```python
from build123d import *

# Parameters (mm, degrees)
F0_W             = 81.28
F0_H             = 58.42
F1_DEPTH         = 3.81
F2_T             = -1.524
F4_DEPTH         = 6.096
F4_COPIES2_COUNT = 2
F6_D             = 1.5113
F6_DEPTH         = 4.826
F6_TIP           = 0.4540403268
F7_R             = 0.635


# Not quite as in the source:
# - a pattern or mirror of a feature is missing from the dataset's text; its kind, count and spacing are read off the source's solid


with BuildPart() as f1:
    # F0 (on Top) → F1 (new body, symmetric)
    with BuildSketch(Plane.XY):
        Rectangle(F0_W, F0_H)
    extrude(amount=F1_DEPTH, both=True)

    # F2
    f2_openings = [f1.faces().sort_by_distance(p)[0] for p in [
        (0, 0, 3.81),
    ]]
    offset(amount=F2_T, openings=f2_openings)

    # F3 (on face) → F4 (join, through all)
    with BuildSketch(Plane.XY.offset(3.81)):
        with BuildLine():
            ThreePointArc((-39.116, 26.162), (-38.0383692655, 26.6083692655), (-37.592, 27.686))
            Line((-37.592, 27.686), (-39.116, 27.686))
            Line((-39.116, 27.686), (-39.116, 26.162))
        make_face()
        with BuildLine():
            ThreePointArc((-13.0386666835, 29.21), (-14.1162974072, 28.7636307286), (-14.5626666667, 27.686))
            Line((-14.5626666667, 27.686), (-11.5146666667, 27.686))
            ThreePointArc((-11.5146666667, 27.686), (-11.9610359381, 28.7636307405), (-13.0386666835, 29.21))
        make_face()
        with BuildLine():
            Line((-39.116, -1.524), (-39.116, 1.524))
            ThreePointArc((-39.116, 1.524), (-40.1936307323, 1.0776307368), (-40.64, 6.4e-09))
            ThreePointArc((-40.64, 6.4e-09), (-40.1936307368, -1.0776307323), (-39.116, -1.524))
        make_face()
        with BuildLine():
            ThreePointArc((14.5626666667, 27.686), (14.1162974012, 28.7636307345), (13.0386666667, 29.21))
            ThreePointArc((13.0386666667, 29.21), (11.9610359321, 28.7636307345), (11.5146666667, 27.686))
            Line((11.5146666667, 27.686), (14.5626666667, 27.686))
        make_face()
        with BuildLine():
            Line((14.5626666667, 27.686), (11.5146666667, 27.686))
            ThreePointArc((11.5146666667, 27.686), (13.0386666667, 26.162), (14.5626666667, 27.686))
        make_face()
        with BuildLine():
            ThreePointArc((-37.592, -27.686), (-38.0383692655, -26.6083692655), (-39.116, -26.162))
            Line((-39.116, -26.162), (-39.116, -27.686))
            Line((-39.116, -27.686), (-37.592, -27.686))
        make_face()
        with BuildLine():
            Line((39.116, 27.686), (37.592, 27.686))
            ThreePointArc((37.592, 27.686), (38.0383692655, 26.6083692655), (39.116, 26.162))
            Line((39.116, 26.162), (39.116, 27.686))
        make_face()
        with BuildLine():
            ThreePointArc((-14.5626666667, -27.686), (-14.1162973989, -28.7636307368), (-13.0386666602, -29.21))
            ThreePointArc((-13.0386666602, -29.21), (-11.9610359299, -28.7636307323), (-11.5146666667, -27.686))
            Line((-11.5146666667, -27.686), (-14.5626666667, -27.686))
        make_face()
        with BuildLine():
            ThreePointArc((11.5146666667, -27.686), (11.9610359295, -28.7636307319), (13.0386666593, -29.21))
            ThreePointArc((13.0386666593, -29.21), (14.1162973986, -28.7636307371), (14.5626666667, -27.686))
            Line((14.5626666667, -27.686), (11.5146666667, -27.686))
        make_face()
        with BuildLine():
            Line((39.116, -1.524), (39.116, 1.524))
            ThreePointArc((39.116, 1.524), (37.592, 0), (39.116, -1.524))
        make_face()
        with BuildLine():
            Line((39.116, -27.686), (39.116, -26.162))
            ThreePointArc((39.116, -26.162), (38.0383692655, -26.6083692655), (37.592, -27.686))
            Line((37.592, -27.686), (39.116, -27.686))
        make_face()
    f4 = extrude(amount=-F4_DEPTH)

    # F4_copies: F4 across plane
    add(f4.mirror(Plane(origin=(0, 0, 0), x_dir=(0, 0, -1), z_dir=(-1, 0, 0))))

    # F4_copies1: F4 across plane
    add(f4.mirror(Plane(origin=(0, 0, 0), x_dir=(0, 0, -1), z_dir=(0, -1, 0))))

    # F4_copies2: F4 ×2 about axis
    f4_copies2_axis = Axis((0, 0, 0), (0, 0, 1))
    for i in range(1, F4_COPIES2_COUNT):
        add(f4.rotate(f4_copies2_axis, i * 360 / F4_COPIES2_COUNT))

    # F6
    with Locations(Plane.XY.offset(3.81)):
        with Locations((-39.116, 27.686), (-13.0386666667, 27.686), (13.0386666667, 27.686), (39.116, 27.686), (39.116, 0), (39.116, -27.686), (13.0386666667, -27.686), (-13.0386666667, -27.686), (-39.116, -27.686), (-39.116, 0)):
            Hole(F6_D / 2, depth=F6_DEPTH)
            with Locations((0, 0, -(F6_DEPTH + F6_TIP / 2))):  # 118° drill point
                Cone(0, F6_D / 2, F6_TIP, mode=Mode.SUBTRACT)

    # F7
    f7_edges = [f1.edges().sort_by_distance(p)[0] for p in [
        (-37.592, 27.686, 0.762),
        (-11.514667, 27.686, 0.762),
        (14.562667, 27.686, 0.762),
        (37.592, 27.686, 0.762),
        (40.64, 0, 0.762),
        (39.116, -26.162, 0.762),
        (37.592, -27.686, 0.762),
        (14.562667, -27.686, 0.762),
        (-11.514667, -27.686, 0.762),
        (-37.592, -27.686, 0.762),
        (39.116, 26.162, 0.762),
        (39.116, 1.524, 0.762),
        (39.116, -1.524, 0.762),
        (11.514667, 27.686, 0.762),
        (11.514667, -27.686, 0.762),
        (-14.562667, 27.686, 0.762),
        (-14.562667, -27.686, 0.762),
        (-39.116, 26.162, 0.762),
        (-39.116, 1.524, 0.762),
        (-39.116, -26.162, 0.762),
        (-39.116, -1.524, 0.762),
    ]]
    fillet(f7_edges, radius=F7_R)


solid = f1.part
```
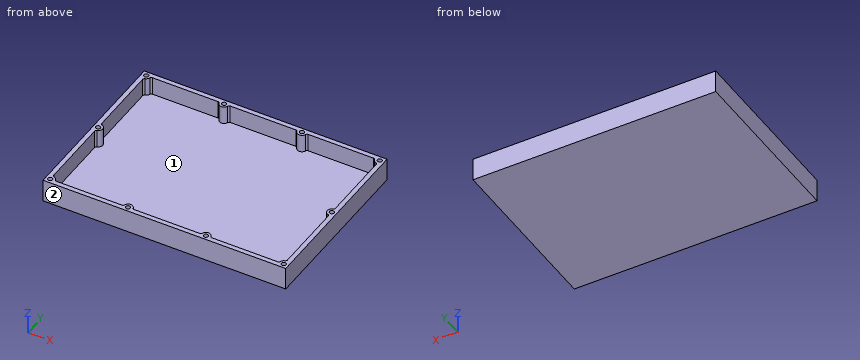
The listing builds one solid part. Answer for the finished solid, in the listing's coordinates (mm). Face numbers are marked on the shaded views. Coordinates: 2 decimals unless noted, no trailing zeros. Write each loop counter-clockwise with the first axis right and the second up, starting at its lowest first coordinate (ties: lowest second). Pieces come first, ordered by that corner, then holes. Notation, with made-up numbers: (4, -19.5) - (26, -19.5) arc R26 ccw to (26, 6.5) - close; hole circle Ø9 at (-28.75, -22). An arc over 180 degrees is marked (long way). One line per item, written item: value.
1) For a pull along X with two mould halves and no side action, classify the marked faces 1 and 2 as pulls with the +X half, pulls with the -X half, needs draft (parallel to the pull), parting line crosses it, or undercut.
Geometry check:
face 1: undercut
face 2: needs draft
2) Find section B-B (x = -29). Give the vertices of the cut face in (y, z).
Geometry check:
outline: (-29.21, -3.81) - (29.21, -3.81) - (29.21, 3.81) - (27.69, 3.81) - (27.69, -2.29) - (-27.69, -2.29) - (-27.69, 3.81) - (-29.21, 3.81) - close
3) Find section A-A (y = -20). Give the vertices of the cut face in (x, z).
Geometry check:
outline: (-40.64, -3.81) - (40.64, -3.81) - (40.64, 3.81) - (39.12, 3.81) - (39.12, -2.29) - (-39.12, -2.29) - (-39.12, 3.81) - (-40.64, 3.81) - close
4) Each of these flat-tipped pins is pushed along its axis until it touches: pin 1 Ø1.4 at (x, y) = (39.116, 27.686) entering from +Z; pin 2 Ø3 at (x, y) = (-6.5, -12) entering from +Z. Where does it stop, or does it pass through?
Geometry check:
pin 1: stops at z = -1.05
pin 2: stops at z = -2.29
5) Find section C-C (z = 0.5). Count the separate pieces of the cut face and the enclosed holes in it, and give its area (3 significant figures).
Geometry check:
separate pieces: 1
enclosed holes: 11
area: 429 mm2
6) Consider line 1 along Y through (x, z) = (13, 3); line 2 along Y through (x, z) = (34, -1.75); line 3 along X through (y, z) = (9, -0.25). Determine where each line is inside the solid, lowest interval first. Write a range as from..to.
Geometry check:
line 1: y = -29.21..-28.44, -26.93..-26.16, 26.16..26.93, 28.44..29.21
line 2: y = -29.21..-27.69, 27.69..29.21
line 3: x = -40.64..-39.12, 39.12..40.64
